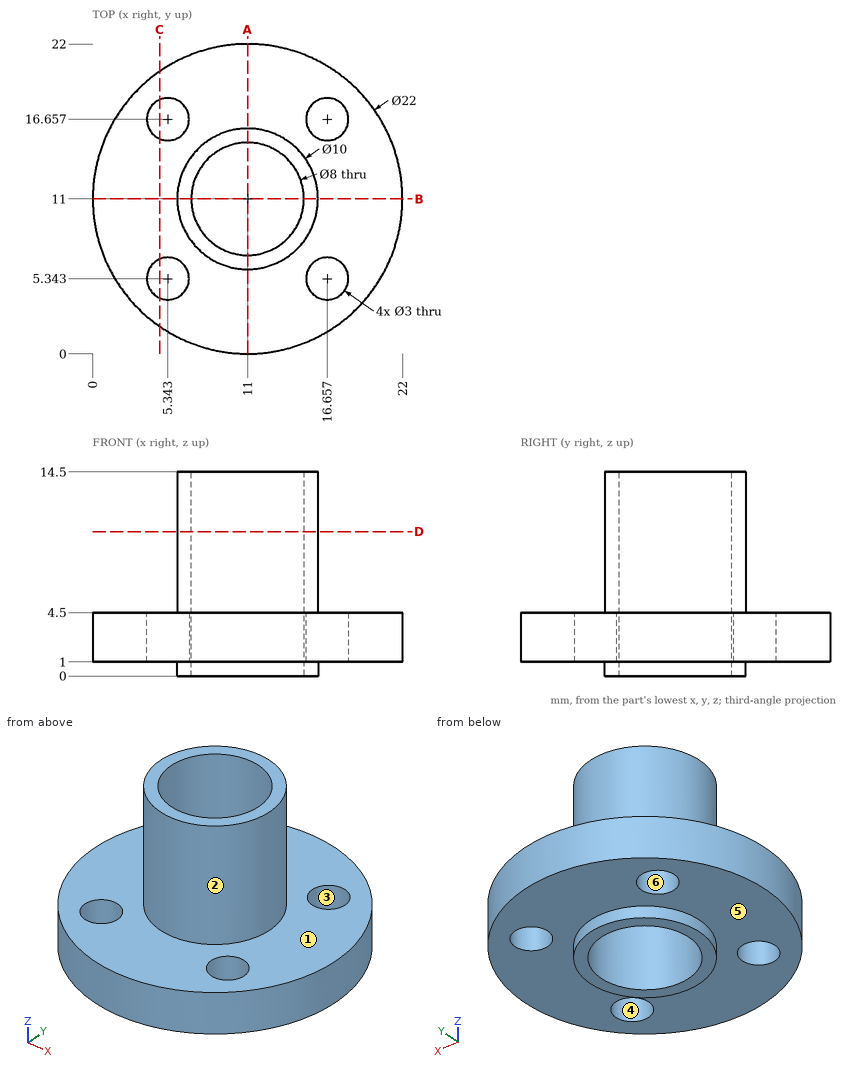
Verification items for this drawing (mm, ordinates from the low corner). A direction names the side the tool comes from. Coordinates: 2 decimals unless noted, no trailing zeros. Order: outer loops, then holes, each group sorted by start corner. A loop starts at its lowest first (then second) coordinate and runs counter-clockwise, first axis right, second up. Notation, with made-up numbers: (-17, 50.25) - (37, 50.25) arc R26 cw to (37, 81.25) - close; hole circle Ø3 at (-0.5, 12.25). An arc over 180 degrees is marked (long way). Use one line per item in the form item = value.
1. Section check A-A (x = 11). Record the boundary of the cut face in (y, z).
Here are the results:
outline = (0, 1) - (6, 1) - (6, 0) - (7, 0) - (7, 14.5) - (6, 14.5) - (6, 4.5) - (0, 4.5) - close; (15, 0) - (16, 0) - (16, 1) - (22, 1) - (22, 4.5) - (16, 4.5) - (16, 14.5) - (15, 14.5) - close
2. Scan lines: line 1 (Y direction, x = 11, z = 6.75); line 2 (X direction, y = 17, z = 4.25); line 3 (Y direction, x = 11, z = 3.5). Record each from-to range of solid material in increasing order.
Here are the results:
line_1 = 6 to 7, 15 to 16
line_2 = 1.78 to 3.88, 6.8 to 15.2, 18.12 to 20.22
line_3 = 0 to 7, 15 to 22
3. Access from +Z, -Z, +X, -X, +Y, -Y to the whole of each face (thin tool, end or side, straight path). Record for the marked faces 5 and 6.
Here are the results:
face_5 = -Z
face_6 = +Z, -Z
4. Draft check along Y on the marked faces 1, 2, 3 and 4. Enter one of: pulls with the +Y half, pulls with the -Y half, needs draft (parallel to the pull), parting line crosses it, or undercut.
Here are the results:
face_1 = needs draft
face_2 = parting line crosses it
face_3 = undercut
face_4 = undercut
5. Section check D-D (z = 10.25). Record the boundary of the cut face in (x, y).
Here are the results:
outline = circle Ø10 at (11, 11); hole circle Ø8 at (11, 11)
6. Gauge pin test, flat ends, axial feed: pin 1 (4 mm diameter, centred on x = 3.5, y = 8, fed in from -Z); pin 2 (7 mm diameter, centred on x = 11, y = 11, fed in from -Z); pin 3 (3 mm diameter, centred on x = 7, y = 4.5, fed in from +Z); pin 4 (3 mm diameter, centred on x = 16, z = 5.5, fed in from +Y). Record the tip position at first contact, or that the pin passes through.
Here are the results:
pin_1 = 1
pin_2 = through
pin_3 = 4.5
pin_4 = 21.29
7. Section check C-C (x = 4.75). Record the boundary of the cut face in (y, z).
Here are the results:
outline = (1.95, 1) - (3.97, 1) - (3.97, 4.5) - (1.95, 4.5) - close; (6.72, 1) - (15.28, 1) - (15.28, 4.5) - (6.72, 4.5) - close; (18.03, 1) - (20.05, 1) - (20.05, 4.5) - (18.03, 4.5) - close
